from build123d import *

# Parameters (mm, degrees)
SKETCH1_R           = 14.3129
BOSS_EXTRUDE1_DEPTH = 3.175
FILLET2_R           = 6.35


with BuildPart() as part:
    # Sketch1 → Boss-Extrude1 (new body)
    with BuildSketch(Plane(origin=(0, 0, 0), x_dir=(1, 0, 0), z_dir=(0, 1, 0))):
        with BuildLine():
            Line((-25.4, 0), (-25.4, -250.825))
            Line((-25.4, -250.825), (141.2875, -250.825))
            Line((141.2875, -250.825), (141.2875, 0))
            Line((141.2875, 0), (25.4, 0))
            ThreePointArc((25.4, 0), (0, 25.4), (-25.4, 0))
        make_face()
        Circle(SKETCH1_R, mode=Mode.SUBTRACT)
    extrude(amount=BOSS_EXTRUDE1_DEPTH)

    # Fillet2
    fillet2_edges = [part.edges().sort_by_distance(p)[0] for p in [
        (25.4, 1.5875, 0),
    ]]
    fillet(fillet2_edges, radius=FILLET2_R)


solid = part.part
Read the model definition and answer for the solid it produces. Units are mm, in the model's axes. Give positions to 0.01 mm unless a question says otherwise; leave off trailing zeros. Write each loop counter-clockwise with the first axis right and the second up, starting at its lowest first coordinate (ties: lowest second). Pieces come first, ordered by that corner, then holes. Notation, with made-up numbers: (38.25, 12) -> (75.25, 12) arc R19 ccw to (75.25, 34) -> close; hole circle Ø11 at (-39, -6). An arc over 180 degrees is marked (long way). Answer as a JSON object with one key per item and string values. Group by question number.
1) Find section D-D (x = 17). Write down the section's boundary in (y, z) (3 decimals), and give its area (3 significant figures).
2) The mould has two halves that part along Z. Classify faces 1 (the cylindrical face through (-1.86, 1.57, -14.19)), 2 (the cylindrical face through (27.045, 1.61, -1.47)), 3 (the flat face through (57, 0, 111)): +Z half, -Z half, draft (parallel to the pull), parting line (faces both ways), or undercut.
3) Consider L1, parallel to Z at x = 0, y = 0.95 (3 decimals); L2, parallel to Z at x = 92, y = 1.9 (3 decimals); L3, parallel to Z at x = 29, y = 0.95 (3 decimals). Determine where each line is inside the solid, lowest interval first. Write a range as from..to.
4) This flat-tipped pin is pushed along its axis until it touches: P1, Ø1, axis at x = 86, y = 1, coming from the -Z side. Where does it stop, or does it pass through?
5) Find section C-C (x = 39). Write down the section's boundary in (y, z) (3 decimals), and give its area (3 significant figures).
6) Find section A-A (x = 0). Write down the section's boundary in (y, z) (3 decimals), and give its area (3 significant figures).
Values follow:
{
 "1": {"outline": "(0, -18.872) -> (3.175, -18.872) -> (3.175, 250.825) -> (0, 250.825) -> close", "area": "856 mm2"},
 "2": {"face 1": "undercut", "face 2": "-Z half", "face 3": "draft"},
 "3": {"L1": "z = -25.4..-14.313, 14.313..250.825", "L2": "z = 0..250.825", "L3": "z = -0.36..250.825"},
 "4": {"P1": "stops at z = 0"},
 "5": {"outline": "(0, 0) -> (3.175, 0) -> (3.175, 250.825) -> (0, 250.825) -> close", "area": "796 mm2"},
 "6": {"outline": "(0, -25.4) -> (3.175, -25.4) -> (3.175, -14.313) -> (0, -14.313) -> close; (0, 14.313) -> (3.175, 14.313) -> (3.175, 250.825) -> (0, 250.825) -> close", "area": "786 mm2"}
}
